Geometry: final body of the model. Coordinates: model frame, mm. A direction names the side the tool comes from. Give positions to 0.01 mm unless a question says otherwise; leave off trailing zeros. Write each loop counter-clockwise with the first axis right and the second up, starting at its lowest first coordinate (ties: lowest second). Pieces come first, ordered by that corner, then holes.
Q1. Draft query along X for faces 1 (the face through (-13.907, -26.547, -13.019)), 2 (the face through (0, -9, 65)), 3 (the face through (-50.99, -7.89, -47.74)), 4 (the face through (-17, 0, -15)). Return one class per face: pulls with the +X half, pulls with the -X half, needs draft (parallel to the pull), parting line crosses it, or undercut.
Q2. Reachability of faces 5 (the face through (-25.589, -36.248, -23.955)), 6 (the face through (-15, -53.848, -14)), 7 (the face through (65, -9, 0)) from +Z, -Z, +X, -X, +Y, -Y: full face, straight path, thin tool, end or side. Return the list, or none.
Q3. Cut plane A-A on y = -5. Return the cut outline in (x, z).
Q4. Cut plane B-B on y = -27.5. Return the cut outline in (x, z), plus the area to 3 significant figures.
Q5. Line query: L1, parallel to Y at x = -63, z = -2; L2, parallel to X at y = -23.5, z = -12; L3, parallel to X at y = -28, z = -17. Output: solid intervals per line, ascending.
Q6. Pin query (flat end, axial travel): pin 1 (2 mm diameter, centred on y = -45, z = -4.5, fed in from -X); pin 2 (10.5 mm diameter, centred on y = -10.5, z = 63.5, fed in from +X); pin 3 (8 mm diameter, centred on x = -40, z = 0.5, fed in from -Y); pin 4 (23 mm diameter, centred on x = 0, z = 0, fed in from -Y). Return the tip coordinate at first contact, or that it passes through.
```python
from build123d import *

# Parameters (mm, degrees)
F0_R     = 35.052
F0_R_2   = 19.05
F1_DEPTH = 53.848
F0_R_3   = 69.85
F2_DEPTH = 19.05
F3_W     = 73.3096525073
F3_H     = 72.7184489369
F4_DEPTH = 222
F5_W     = 74.8862102628
F5_H     = 75.4774138331
F6_DEPTH = 53.849
F7_R     = 3.048


# Not quite as in the source:
# - an extrude ends at something that could not be found from the text; its depth is read off the source's solid


with BuildPart() as f1:
    # F0 (on Front) → F1 (new body)
    with BuildSketch(Plane.XZ):
        Circle(F0_R)
        Circle(F0_R_2, mode=Mode.SUBTRACT)
    extrude(amount=F1_DEPTH)

    # F0 (on Front) → F2 (join)
    with BuildSketch(Plane.XZ):
        Circle(F0_R_3)
        with BuildLine():
            ThreePointArc((6.3389523479, 53.4735896226), (38.0762859533, 38.0762859533), (53.4735896226, 6.3389523479))
            ThreePointArc((53.4735896226, 6.3389523479), (58.2037429965, 4.6206063399), (60.198, 0))
            ThreePointArc((60.198, 0), (58.2037429965, -4.6206063399), (53.4735896226, -6.3389523479))
            ThreePointArc((53.4735896226, -6.3389523479), (38.0762859533, -38.0762859533), (6.3389523479, -53.4735896226))
            ThreePointArc((6.3389523479, -53.4735896226), (6.3472374861, -53.6607133338), (6.35, -53.848))
            ThreePointArc((6.35, -53.848), (-0.1872866662, -60.1952374861), (-6.3389523479, -53.4735896226))
            ThreePointArc((-6.3389523479, -53.4735896226), (-38.0762859533, -38.0762859533), (-53.4735896226, -6.3389523479))
            ThreePointArc((-53.4735896226, -6.3389523479), (-60.198, 0), (-53.4735896226, 6.3389523479))
            ThreePointArc((-53.4735896226, 6.3389523479), (-38.0762859533, 38.0762859533), (-6.3389523479, 53.4735896226))
            ThreePointArc((-6.3389523479, 53.4735896226), (-0.1872866662, 60.1952374861), (6.35, 53.848))
            ThreePointArc((6.35, 53.848), (6.3472374861, 53.6607133338), (6.3389523479, 53.4735896226))
        make_face(mode=Mode.SUBTRACT)
        with BuildLine():
            ThreePointArc((53.4735896226, -6.3389523479), (47.498, 0), (53.4735896226, 6.3389523479))
            ThreePointArc((53.4735896226, 6.3389523479), (38.0762859533, 38.0762859533), (6.3389523479, 53.4735896226))
            ThreePointArc((6.3389523479, 53.4735896226), (0, 47.498), (-6.3389523479, 53.4735896226))
            ThreePointArc((-6.3389523479, 53.4735896226), (-38.0762859533, 38.0762859533), (-53.4735896226, 6.3389523479))
            ThreePointArc((-53.4735896226, 6.3389523479), (-49.2273936601, 4.3557429965), (-47.498, 0))
            ThreePointArc((-47.498, 0), (-49.2273936601, -4.3557429965), (-53.4735896226, -6.3389523479))
            ThreePointArc((-53.4735896226, -6.3389523479), (-38.0762859533, -38.0762859533), (-6.3389523479, -53.4735896226))
            ThreePointArc((-6.3389523479, -53.4735896226), (0, -47.498), (6.3389523479, -53.4735896226))
            ThreePointArc((6.3389523479, -53.4735896226), (38.0762859533, -38.0762859533), (53.4735896226, -6.3389523479))
        make_face()
        Circle(F0_R, mode=Mode.SUBTRACT)
    extrude(amount=F2_DEPTH)

    # F3 (on Front) → F4 (cut, through all)
    with BuildSketch(Plane.XZ):
        with Locations((36.6548262537, 36.3592244685)):
            Rectangle(F3_W, F3_H)
    extrude(amount=-F4_DEPTH, mode=Mode.SUBTRACT)

    # F5 (on Front) → F6 (cut, through all)
    with BuildSketch(Plane.XZ):
        with Locations((37.4431051314, 37.7387069166)):
            Rectangle(F5_W, F5_H)
    extrude(amount=F6_DEPTH, mode=Mode.SUBTRACT)

    # F7
    f7_edges = [f1.edges().sort_by_distance(p)[0] for p in [
        (-24.785507, -53.848, -24.785507),
        (-24.785507, -19.05, -24.785507),
        (-49.391409, -19.05, -49.391409),
    ]]
    fillet(f7_edges, radius=F7_R)


solid = f1.part
```
Data:
1. face 1: undercut
1. face 2: pulls with the +X half
1. face 3: parting line crosses it
1. face 4: needs draft
2. face 5: -Y
2. face 6: +Z, -Z, +X, -X, -Y
2. face 7: +Z, +X, +Y, -Y
3. outline: (0, 19.05) - (0, 47.5) arc R6.35 cw to (0, 60.2) - (0, 69.85) arc R69.85 ccw (long way) to (69.85, 0) - (60.2, 0) arc R6.35 cw to (47.5, 0) - (19.05, 0) arc R19.05 cw (long way) to start; hole circle Ø12.7 at (-53.85, 0); hole circle Ø12.7 at (0, -53.85)
4. outline: (0, 19.05) - (0, 35.05) arc R35.05 ccw (long way) to (35.05, 0) - (19.05, 0) arc R19.05 cw (long way) to start
4. area: 2,040 mm2
5. L1: y = -19.05 to 0
5. L2: x = -32.93 to -14.8, 14.8 to 32.93
5. L3: x = -30.65 to -8.6, 8.6 to 30.65
6. pin 1: stops at x = -34.88
6. pin 2: stops at x = 0
6. pin 3: stops at y = -19.89
6. pin 4: passes through
